from build123d import *

# Parameters (mm, degrees)
F0_R     = 20
F1_DEPTH = 700
F2_R     = 40
F2_R_2   = 3
F3_DEPTH = 2


with BuildPart() as f1:
    # F0 (on Top) → F1 (new body)
    with BuildSketch(Plane.XY):
        Circle(F0_R)
    extrude(amount=-F1_DEPTH)

    # F2 (on Top) → F3 (join)
    with BuildSketch(Plane.XY):
        Circle(F2_R)
        with Locations((-1.2432069331, -30)):
            Circle(F2_R_2, mode=Mode.SUBTRACT)
        with Locations((-30, 0)):
            Circle(F2_R_2, mode=Mode.SUBTRACT)
        with Locations((-1.2432069331, 30)):
            Circle(F2_R_2, mode=Mode.SUBTRACT)
        with Locations((28.7567930669, 0)):
            Circle(F2_R_2, mode=Mode.SUBTRACT)
    extrude(amount=F3_DEPTH)


solid = f1.part
Here's how the part is built. I have some questions about the finished solid (model axes, mm). A direction names the side the tool comes from. Coordinates: 2 decimals unless noted, no trailing zeros. Order: outer loops, then holes, each group sorted by start corner. A loop starts at its lowest first (then second) coordinate and runs counter-clockwise, first axis right, second up. Notation, with made-up numbers: (53.5, 63) -> (93.5, 63) arc R18 ccw to (93.5, 68) -> close; hole circle Ø3 at (83, -16.75). An arc over 180 degrees is marked (long way). Answer in a Markdown table with one row per item.
(1) Will these pins go through, and if not, where does the flat tip stop? pin 1 Ø6 at (x, z) = (-18.5, -416) entering from +Y; pin 2 Ø4 at (x, z) = (20.5, -383) entering from +Y; pin 3 Ø5 at (x, y) = (14, -20.5) entering from -Z; pin 4 Ø3.5 at (x, y) = (-1.24, -30) entering from +Z.
Answer key:
| item | result |
|---|---|
| pin 1 | y = 12.64 |
| pin 2 | y = 7.6 |
| pin 3 | z = 0 |
| pin 4 | through |
(2) I want a section at A-A on y = -12.5. List the corners of the cut face in (x, z) for me.
Answer key:
| item | result |
|---|---|
| outline | (-38, 0) -> (-15.61, 0) -> (-15.61, -700) -> (15.61, -700) -> (15.61, 0) -> (38, 0) -> (38, 2) -> (-38, 2) -> close |
(3) I want a section at C-C on x = -10.5. List the corners of the cut face in (y, z) for me.
Answer key:
| item | result |
|---|---|
| outline | (-38.6, 0) -> (-17.02, 0) -> (-17.02, -700) -> (17.02, -700) -> (17.02, 0) -> (38.6, 0) -> (38.6, 2) -> (-38.6, 2) -> close |
(4) Please list where these lines run through material, in increasing order: probe 1 along Z at (x, y) = (-27, 27); probe 2 along X at (y, z) = (-17, -664); probe 3 along Y at (x, z) = (9.5, -89.5).
Answer key:
| item | result |
|---|---|
| probe 1 | 0 to 2 |
| probe 2 | -10.54 to 10.54 |
| probe 3 | -17.6 to 17.6 |
(5) I want a section at B-B on z = -419. List the corners of the cut face in (x, y) for me.
Answer key:
| item | result |
|---|---|
| outline | circle Ø40 at (0, 0) |
(6) On a 3-axis mill with a long thin cutter (end or side, diameter ignored), from which of +Z, -Z, +X, -X, +Y, -Y can I reach the whole of each face in a straight line? I mean faces 1 (the face through (-4.336, -19.524, -345.1)), 2 (the face through (-8.67, -39.05, 0.99)). Say none if no direction works.
Answer key:
| item | result |
|---|---|
| face 1 | -Z |
| face 2 | +Z, -Z |
